Job drawing, mm, ordinate dimensions from the low corner. One solid piece. A direction names the side the tool comes from. Give positions to 0.01 mm unless a question says otherwise; leave off trailing zeros. Loops run counter-clockwise (first coordinate to the right, second up) from the corner with the lowest first, then second, coordinate; pieces in that order, holes last. Notation, with made-up numbers: M 85,62.25 L 136,62.25 A35 cw 136,98.25 Z; hole C 64.25,-20 d9. An arc over 180 degrees is marked long. Answer as CSV lines item,"result".
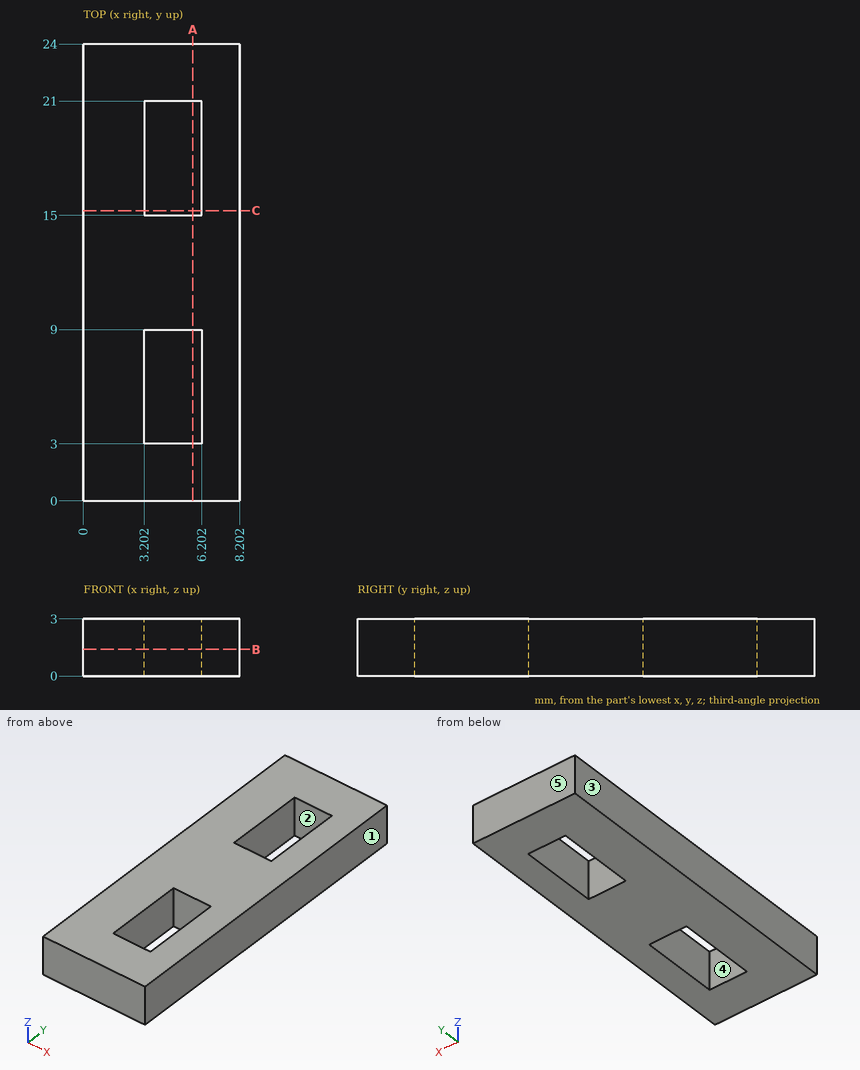
1) Drill centre lines: line 1 (Y direction, x = 5, z = 2.6); line 2 (X direction, y = 6, z = 0.25). Where is each one in solid material? Low to high. Write a range as from..to.
Answer below:
line 1,"y = 0..3, 9..15, 21..24"
line 2,"x = 0..3.2, 6.2..8.2"
2) Mould opens along X. For the marked faces 1, 2 and 3 say: +X half, -X half, draft (parallel to the pull), parting line (faces both ways), or undercut.
Answer below:
face 1,"+X half"
face 2,"undercut"
face 3,"-X half"
3) Band-saw the part on B-B on z = 1.4. Give the cut face in (x, y), and give its area (3 significant figures).
Answer below:
outline,"M 0,0 L 8.2,0 L 8.2,24 L 0,24 Z; hole M 3.2,3 L 6.2,3 L 6.2,9 L 3.2,9 Z; hole M 3.2,15 L 6.2,15 L 6.2,21 L 3.2,21 Z"
area,"161 mm^2"
4) Band-saw the part on C-C on y = 15.25. Give the cut face in (x, z), and give its area (3 significant figures).
Answer below:
outline,"M 0,0 L 3.2,0 L 3.2,3 L 0,3 Z; M 6.2,0 L 8.2,0 L 8.2,3 L 6.2,3 Z"
area,"15.6 mm^2"
5) Band-saw the part on A-A on x = 5.75. Give the cut face in (y, z), and give its area (3 significant figures).
Answer below:
outline,"M 0,0 L 3,0 L 3,3 L 0,3 Z; M 9,0 L 15,0 L 15,3 L 9,3 Z; M 21,0 L 24,0 L 24,3 L 21,3 Z"
area,"36.0 mm^2"
6) Which spindle directions (+Z, -Z, +X, -X, +Y, -Y) get a long thin tool onto all of the face, cutting with end or side? Do the marked faces 4 and 5. Say none if no direction does.
Answer below:
face 4,"+Z, -Z"
face 5,"+Z, -Z, +X, -X, +Y"
